from build123d import *

# Parameters (mm, degrees)
F1_DEPTH = 510.54
F2_W     = 25.4
F2_H     = 76.2
F3_DEPTH = 76.2
F4_R     = 31.75


with BuildPart() as f1:
    # F0 (on Top) → F1 (new body)
    with BuildSketch(Plane.XY):
        with BuildLine():
            Line((297.18, 685.8), (-297.18, 685.8))
            Line((-297.18, 685.8), (-297.18, 0))
            ThreePointArc((-297.18, 0), (0, 25.4), (297.18, 0))
            Line((297.18, 0), (297.18, 685.8))
        make_face()
    extrude(amount=F1_DEPTH)

    # F2 (on face) → F3 (join)
    with BuildSketch(Plane(origin=(0, 685.8, 0), x_dir=(-1, 0, 0), z_dir=(0, 1, 0))):
        with Locations((-265.43, 459.74)):
            Rectangle(F2_W, F2_H)
        with Locations((265.43, 459.74)):
            Rectangle(F2_W, F2_H)
        with Locations((-265.43, 50.8)):
            Rectangle(F2_W, F2_H)
        with Locations((265.43, 50.8)):
            Rectangle(F2_W, F2_H)
    extrude(amount=F3_DEPTH)

    # F4
    f4_edges = [f1.edges().sort_by_distance(p)[0] for p in [
        (265.43, 762, 497.84),
        (265.43, 762, 421.64),
        (265.43, 762, 88.9),
        (-265.43, 762, 12.7),
        (-265.43, 762, 88.9),
        (-265.43, 762, 421.64),
        (-265.43, 762, 497.84),
        (265.43, 762, 12.7),
    ]]
    fillet(f4_edges, radius=F4_R)


solid = f1.part
Could you check a few things on this model? Use its own coordinates, in mm. A direction names the side the tool comes from. Give positions to 0.01 mm unless a question says otherwise; leave off trailing zeros. Write each loop counter-clockwise with the first axis right and the second up, starting at its lowest first coordinate (ties: lowest second). Pieces come first, ordered by that corner, then holes. Notation, with made-up numbers: (57, 17.25) -> (98, 17.25) arc R16 ccw to (98, 41.25) -> close; hole circle Ø7 at (27.5, 56). An arc over 180 degrees is marked (long way). Answer as a JSON object with one key per item and string values.
Q1. Which directions (+Z, -Z, +X, -X, +Y, -Y) give clear straight access to the entire face, cutting with the end or side of a thin tool? Please do faces 1 (the flat face through (278.13, 723, 50)), 2 (the flat face through (-252.73, 723, 50)), 3 (the cylindrical face through (-265.61, 752.45, 430.69)).
Taken from the geometry:
{"face 1": "+Z, -Z, +X, +Y", "face 2": "+Z, -Z, +Y", "face 3": "+X, -X, +Y"}
Q2. Will these pins go through, and if not, where does the flat tip stop? pin 1 Ø2 at (x, z) = (201, 443) entering from -Y; pin 2 Ø12.5 at (x, y) = (266.5, 713.5) entering from +Z; pin 3 Ø7.5 at (x, y) = (266.5, 701.5) entering from -Z.
Taken from the geometry:
{"pin 1": "stops at y = 13.71", "pin 2": "stops at z = 497.84", "pin 3": "stops at z = 12.7"}
Q3. Suppose I cut it at C-C on z = 75.5. Write out the boundary of the cut face in (x, y), then the cut area to 3 significant figures.
Taken from the geometry:
{"outline": "(-297.18, 0) arc R1751.2 cw to (297.18, 0) -> (297.18, 685.8) -> (278.13, 685.8) -> (278.13, 756.16) -> (252.73, 756.16) -> (252.73, 685.8) -> (-252.73, 685.8) -> (-252.73, 756.16) -> (-278.13, 756.16) -> (-278.13, 685.8) -> (-297.18, 685.8) -> close", "area": "401,000 mm²"}
Q4. Suppose I cut it at B-B on x = 93. Write out the boundary of the cut face in (y, z).
Taken from the geometry:
{"outline": "(22.93, 0) -> (685.8, 0) -> (685.8, 510.54) -> (22.93, 510.54) -> close"}
Q5. Suppose I cut it at D-D on z = 478. Write out the boundary of the cut face in (x, y), then the cut area to 3 significant figures.
Taken from the geometry:
{"outline": "(-297.18, 0) arc R1751.2 cw to (297.18, 0) -> (297.18, 685.8) -> (278.13, 685.8) -> (278.13, 759.68) -> (252.73, 759.68) -> (252.73, 685.8) -> (-252.73, 685.8) -> (-252.73, 759.68) -> (-278.13, 759.68) -> (-278.13, 685.8) -> (-297.18, 685.8) -> close", "area": "401,000 mm²"}
Q6. Suppose I cut it at A-A on z = 356. Write out the boundary of the cut face in (x, y).
Taken from the geometry:
{"outline": "(-297.18, 0) arc R1751.2 cw to (297.18, 0) -> (297.18, 685.8) -> (-297.18, 685.8) -> close"}
Q7. Please list where these lines run through material, in increasing order: L1, parallel to X at y = 712, z = 49; L2, parallel to Y at x = -9, z = 400; L3, parallel to Y at x = -149, z = 356.
Taken from the geometry:
{"L1": "x = -278.13 to -252.73, 252.73 to 278.13", "L2": "y = 25.38 to 685.8", "L3": "y = 19.05 to 685.8"}
